from build123d import *

# Parameters (mm, degrees)
F0_W     = 60
F0_H     = 75
F1_DEPTH = 10
F2_R     = 3.25
F3_DEPTH = 10.001
F5_DEPTH = 6


with BuildPart() as f1:
    # F0 (on Top) → F1 (new body)
    with BuildSketch(Plane.XY):
        Rectangle(F0_W, F0_H)
    extrude(amount=-F1_DEPTH)

    # F2 (on Top) → F3 (cut, through all)
    with BuildSketch(Plane.XY):
        with Locations((-23.5, 30)):
            Circle(F2_R)
        with Locations((23.5, 30)):
            Circle(F2_R)
        with Locations((-23.5, -30)):
            Circle(F2_R)
        with Locations((23.5, -30)):
            Circle(F2_R)
    extrude(amount=-F3_DEPTH, mode=Mode.SUBTRACT)

    # F4 (on face) → F5 (cut)
    with BuildSketch(Plane.XY):
        with BuildLine():
            Line((-30, 3), (-30, 0))
            Line((-30, 0), (-30, -3))
            Line((-30, -3), (-26.833333, -3))
            Line((-26.833333, -3), (-26, -3))
            Line((-26, -3), (-16.833333, -3))
            ThreePointArc((-16.833333, -3), (-15.951367, -2.263932), (-14.833333, -2))
            Line((-14.833333, -2), (-6.5, -2))
            ThreePointArc((-6.5, -2), (-5.381966, -2.263932), (-4.5, -3))
            Line((-4.5, -3), (-2.257359, -3))
            Line((-2.257359, -3), (2.257359, -3))
            Line((2.257359, -3), (4.5, -3))
            ThreePointArc((4.5, -3), (5.381966, -2.263932), (6.5, -2))
            Line((6.5, -2), (14.833333, -2))
            ThreePointArc((14.833333, -2), (15.951367, -2.263932), (16.833333, -3))
            Line((16.833333, -3), (26, -3))
            Line((26, -3), (26.833333, -3))
            Line((26.833333, -3), (30, -3))
            Line((30, -3), (30, 0))
            Line((30, 0), (30, 3))
            Line((30, 3), (26.833333, 3))
            Line((26.833333, 3), (26, 3))
            Line((26, 3), (25.333333, 3.5))
            Line((25.333333, 3.5), (19.2, 8.1))
            Line((19.2, 8.1), (9.2, 15.6))
            ThreePointArc((9.2, 15.6), (7.923025, 16.269075), (6.5, 16.5))
            Line((6.5, 16.5), (0, 16.5))
            Line((0, 16.5), (-6.5, 16.5))
            ThreePointArc((-6.5, 16.5), (-7.923025, 16.269075), (-9.2, 15.6))
            Line((-9.2, 15.6), (-19.2, 8.1))
            Line((-19.2, 8.1), (-25.333333, 3.5))
            Line((-25.333333, 3.5), (-26, 3))
            Line((-26, 3), (-26.833333, 3))
            Line((-26.833333, 3), (-30, 3))
        make_face()
        with BuildLine():
            ThreePointArc((-14.833333, 2), (-15.951367, 2.263932), (-16.833333, 3))
            ThreePointArc((-16.833333, 3), (-17.308207, 4.853553), (-16.333333, 6.5))
            Line((-16.333333, 6.5), (-8, 12.75))
            ThreePointArc((-8, 12.75), (-5.381966, 12.986068), (-4, 10.75))
            Line((-4, 10.75), (-4, 4.5))
            ThreePointArc((-4, 4.5), (-4.128292, 3.709431), (-4.5, 3))
            ThreePointArc((-4.5, 3), (-5.381966, 2.263932), (-6.5, 2))
            Line((-6.5, 2), (-14.833333, 2))
        make_face(mode=Mode.SUBTRACT)
        with BuildLine():
            ThreePointArc((6.5, 2), (5.381966, 2.263932), (4.5, 3))
            ThreePointArc((4.5, 3), (4.128292, 3.709431), (4, 4.5))
            Line((4, 4.5), (4, 10.75))
            ThreePointArc((4, 10.75), (5.381966, 12.986068), (8, 12.75))
            Line((8, 12.75), (16.333333, 6.5))
            ThreePointArc((16.333333, 6.5), (17.205042, 3.709431), (14.833333, 2))
            Line((14.833333, 2), (6.5, 2))
        make_face(mode=Mode.SUBTRACT)
        with BuildLine():
            ThreePointArc((-25.333333, 3.5), (-26.042764, 3.128292), (-26.833333, 3))
            Line((-26.833333, 3), (-26, 3))
            Line((-26, 3), (-25.333333, 3.5))
        make_face()
        with BuildLine():
            Line((-26, -3), (-26.833333, -3))
            ThreePointArc((-26.833333, -3), (-26.042764, -3.128292), (-25.333333, -3.5))
            Line((-25.333333, -3.5), (-26, -3))
        make_face()
        with BuildLine():
            Line((-16.833333, -3), (-26, -3))
            Line((-26, -3), (-25.333333, -3.5))
            Line((-25.333333, -3.5), (-19.2, -8.1))
            Line((-19.2, -8.1), (-9.2, -15.6))
            ThreePointArc((-9.2, -15.6), (-7.923025, -16.269075), (-6.5, -16.5))
            Line((-6.5, -16.5), (0, -16.5))
            Line((0, -16.5), (6.5, -16.5))
            ThreePointArc((6.5, -16.5), (7.923025, -16.269075), (9.2, -15.6))
            Line((9.2, -15.6), (19.2, -8.1))
            Line((19.2, -8.1), (25.333333, -3.5))
            Line((25.333333, -3.5), (26, -3))
            Line((26, -3), (16.833333, -3))
            ThreePointArc((16.833333, -3), (17.308207, -4.853553), (16.333333, -6.5))
            Line((16.333333, -6.5), (8, -12.75))
            ThreePointArc((8, -12.75), (5.381966, -12.986068), (4, -10.75))
            Line((4, -10.75), (4, -4.5))
            ThreePointArc((4, -4.5), (4.128292, -3.709431), (4.5, -3))
            Line((4.5, -3), (2.257359, -3))
            Line((2.257359, -3), (-2.257359, -3))
            Line((-2.257359, -3), (-4.5, -3))
            ThreePointArc((-4.5, -3), (-4.128292, -3.709431), (-4, -4.5))
            Line((-4, -4.5), (-4, -10.75))
            ThreePointArc((-4, -10.75), (-5.381966, -12.986068), (-8, -12.75))
            Line((-8, -12.75), (-16.333333, -6.5))
            ThreePointArc((-16.333333, -6.5), (-17.308207, -4.853553), (-16.833333, -3))
        make_face()
        with BuildLine():
            Line((26.833333, -3), (26, -3))
            Line((26, -3), (25.333333, -3.5))
            ThreePointArc((25.333333, -3.5), (26.042764, -3.128292), (26.833333, -3))
        make_face()
        with BuildLine():
            ThreePointArc((26.833333, 3), (26.042764, 3.128292), (25.333333, 3.5))
            Line((25.333333, 3.5), (26, 3))
            Line((26, 3), (26.833333, 3))
        make_face()
    extrude(amount=-F5_DEPTH, mode=Mode.SUBTRACT)


solid = f1.part
Can you work these out from the model? Positions are in its coordinate system, mm. A direction names the side the tool comes from. Coordinates: 2 decimals unless noted, no trailing zeros. Write each loop counter-clockwise with the first axis right and the second up, starting at its lowest first coordinate (ties: lowest second). Pieces come first, ordered by that corner, then holes. Notation, with made-up numbers: (62, 87.5) - (103, 87.5) arc R22 cw to (103, 118.5) - close; hole circle Ø7 at (32.5, 44). An arc over 180 degrees is marked (long way). Return JSON: item names as keys, results as strings. Group by question number.
Item 1: Which directions (+Z, -Z, +X, -X, +Y, -Y) give clear straight access to the entire face, cutting with the end or side of a thin tool? Please do faces 4 (the face through (11, 2, -3)), 5 (the face through (-28, -3, -3)), 6 (the face through (28, -3, -3)), 7 (the face through (7.904, -16.275, -2.958)), 8 (the face through (9, -6, 0)).
Item 2: I'm going to push a flat-ended pin straight in: pin 1 Ø5 at (x, y) = (-23.5, 30) entering from +Z. Where does the tip first touch, or does it pass through?
Item 3: If we section it at B-B (x = -2): Write out the boundary of the cut face in (y, z), then the cut area to 3 significant figures.
Item 4: We'd pull the mould along Y, two halves only. Please class faces 1 (the face through (12.108, 9.669, -2.958)), 2 (the face through (4, -8, -3)), 3 (the face through (0, 1, -10)): pulls with the +Y half, pulls with the -Y half, needs draft (parallel to the pull), parting line crosses it, or undercut.
Item 5: If we section it at C-C (x = 23.5): Write out the boundary of the cut face in (y, z) (3 decimals), then the cut area to 4 significant figures.
Item 6: If we section it at D-D (z = -2.25): Count the separate pieces of the cut face and the enclosed holes in it, then the cut area to 3 significant figures.
Item 7: If we section it at A-A (y = 30): Write out the boundary of the cut face in (x, z), then the cut area to 3 significant figures.
Item 8: Please list where these lines run through material, in increasing order: probe 1 along Y at (x, z) = (23.5, -7.75); probe 2 along Y at (x, z) = (15.5, -5.75) (3 decimals); probe 3 along Y at (x, z) = (-23.5, -5) (3 decimals).
Return value:
{
 "1": {"face 4": "+Z, +X, -X", "face 5": "+Z, -X", "face 6": "+Z, +X", "face 7": "+Z", "face 8": "+Z, +X, -X, +Y, -Y"},
 "2": {"pin 1": "passes through"},
 "3": {"outline": "(-37.5, -10) - (37.5, -10) - (37.5, 0) - (16.5, 0) - (16.5, -6) - (-16.5, -6) - (-16.5, 0) - (-37.5, 0) - close", "area": "552 mm^2"},
 "4": {"face 1": "undercut", "face 2": "undercut", "face 3": "needs draft"},
 "5": {"outline": "(-37.5, -10) - (-33.25, -10) - (-33.25, 0) - (-37.5, 0) - close; (-26.75, -10) - (26.75, -10) - (26.75, 0) - (4.875, 0) - (4.875, -6) - (-4.875, -6) - (-4.875, 0) - (-26.75, 0) - close; (33.25, -10) - (37.5, -10) - (37.5, 0) - (33.25, 0) - close", "area": "561.5 mm^2"},
 "6": {"separate pieces": "6", "enclosed holes": "4", "area": "3,520 mm^2"},
 "7": {"outline": "(-30, -10) - (-26.75, -10) - (-26.75, 0) - (-30, 0) - close; (-20.25, -10) - (20.25, -10) - (20.25, 0) - (-20.25, 0) - close; (26.75, -10) - (30, -10) - (30, 0) - (26.75, 0) - close", "area": "470 mm^2"},
 "8": {"probe 1": "y = -37.5 to -33.25, -26.75 to 26.75, 33.25 to 37.5", "probe 2": "y = -37.5 to -10.875, -7.125 to -2.091, 2.091 to 7.125, 10.875 to 37.5", "probe 3": "y = -37.5 to -33.25, -26.75 to -4.875, 4.875 to 26.75, 33.25 to 37.5"}
}
